The listing builds one solid part. Answer for the finished solid, in the listing's coordinates (mm). Face numbers are marked on the shaded views. A direction names the side the tool comes from. Give positions to 0.01 mm unless a question says otherwise; leave off trailing zeros. Order: outer loops, then holes, each group sorted by start corner. A loop starts at its lowest first (then second) coordinate and runs counter-clockwise, first axis right, second up.
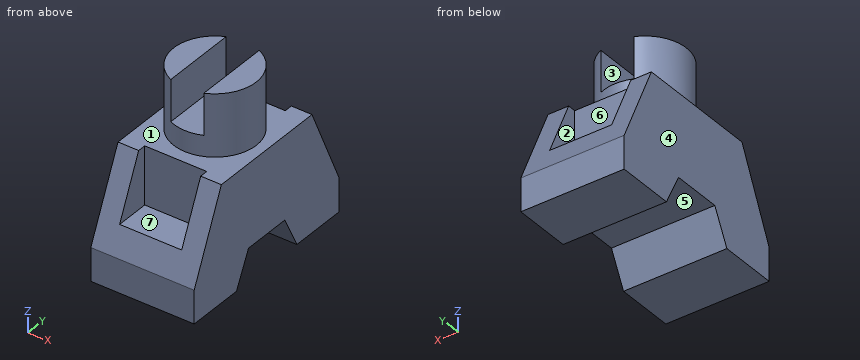
```python
from build123d import *

# Parameters (mm, degrees)
F0_W     = 9
F0_H     = 8
F0_W_2   = 5
F0_H_2   = 18
F0_W_3   = 10
F0_H_3   = 2
F1_DEPTH = 12.5
F2_R     = 10
F3_DEPTH = 15
F5_DEPTH = 10
F6_W     = 15
F6_H     = 8.3
F7_DEPTH = 14


with BuildPart() as f1:
    # F0 (on Right) → F1 (new body, symmetric)
    with BuildSketch(Plane.YZ):
        with Locations((-19.5, -10)):
            Rectangle(F0_W, F0_H)
        Polygon((-15, -6), (-15, -4), (-23.1, -4), (-24, -6), align=None)
        Polygon((-15, -4), (-15, 14), (-23.1, -4), align=None)
        with Locations((-12.5, 5)):
            Rectangle(F0_W_2, F0_H_2)
        with Locations((-7.5, 5)):
            Rectangle(F0_W_2, F0_H_2)
        with Locations((0, 5)):
            Rectangle(F0_W_3, F0_H_2)
        with Locations((7.5, 5)):
            Rectangle(F0_W_2, F0_H_2)
        with Locations((12.5, 5)):
            Rectangle(F0_W_2, F0_H_2)
        Polygon((23.1, -4), (15, 14), (15, -4), align=None)
        Polygon((23.1, -4), (15, -4), (15, -6), (24, -6), align=None)
        with Locations((19.5, -10)):
            Rectangle(F0_W, F0_H)
        with Locations((12.5, -10)):
            Rectangle(F0_W_2, F0_H)
        Polygon((10, -14), (10, -6), (6, -6), align=None)
        with Locations((12.5, -5)):
            Rectangle(F0_W_2, F0_H_3)
        with Locations((0, -5)):
            Rectangle(F0_W_3, F0_H_3)
        Polygon((-5, -6), (-5, -4), (-6, -6), align=None)
        Polygon((6, -6), (5, -4), (5, -6), align=None)
        Polygon((10, -6), (10, -4), (5, -4), (6, -6), align=None)
        Polygon((-6, -6), (-5, -4), (-10, -4), (-10, -6), align=None)
        Polygon((-10, -14), (-6, -6), (-10, -6), align=None)
        with Locations((-12.5, -10)):
            Rectangle(F0_W_2, F0_H)
        with Locations((-12.5, -5)):
            Rectangle(F0_W_2, F0_H_3)
    extrude(amount=F1_DEPTH, both=True)

    # F2 (on face) → F3 (join)
    with BuildSketch(Plane.XY.offset(14)):
        Circle(F2_R)
    extrude(amount=F3_DEPTH)

    # F4 (on face) → F5 (cut)
    with BuildSketch(Plane.XY.offset(29)):
        with BuildLine():
            ThreePointArc((4, 9.1651513899), (2.0430964369, 9.7890631293), (0, 10))
            ThreePointArc((0, 10), (-2.0430964369, 9.7890631293), (-4, 9.1651513899))
            Line((-4, 9.1651513899), (-4, -9.1651513899))
            ThreePointArc((-4, -9.1651513899), (-2.0430964369, -9.7890631293), (0, -10))
            ThreePointArc((0, -10), (2.0430964369, -9.7890631293), (4, -9.1651513899))
            Line((4, -9.1651513899), (4, 9.1651513899))
        make_face()
    extrude(amount=-F5_DEPTH, mode=Mode.SUBTRACT)

    # F6 (on Top) → F7 (cut)
    with BuildSketch(Plane.XY):
        with Locations((0, -17.15)):
            Rectangle(F6_W, F6_H)
        with Locations((0, 17.15)):
            Rectangle(F6_W, F6_H)
    extrude(amount=F7_DEPTH, mode=Mode.SUBTRACT)


solid = f1.part
```
1) Straight lines are drawn through the part: probe 1 along Z at (x, y) = (10.25, -11.5); probe 2 along Y at (x, z) = (2.5, -6.5); probe 3 along Y at (x, z) = (0.25, 5). For each, find the intervals that lie inside material, in ascending order.
Geometry says:
probe 1: z = -14 to 14
probe 2: y = -24 to -6.25, 6.25 to 24
probe 3: y = -13 to 13
2) Find section D-D (z = 26). Write down the section's boundary in (x, y).
Geometry says:
outline: (-4, -9.17) - (-4, 9.17) arc R10 ccw to start; (4, -9.17) arc R10 ccw to (4, 9.17) - close
3) For a pull along X with two mould halves and no side action, classify the marked faces 4, 5, 6 and 7 as +X half, -X half, draft (parallel to the pull), parting line (faces both ways), or undercut.
Geometry says:
face 4: -X half
face 5: draft
face 6: undercut
face 7: undercut
4) A tool of negligible diameter and unlimited length cuts with its end or side. For the marked faces 1, 2 and 3, from which of +Z, -Z, +X, -X, +Y, -Y can it reach the whole face along a straight path? Write none if from no direction.
Geometry says:
face 1: +Z
face 2: +Z, +Y
face 3: +Z, +Y, -Y
5) Given P1, Ø9.5, axis at x = 2, y = -3, coming from the -Z side; P2, Ø1, axis at y = -9, z = 20, coming from the +X side; P3, Ø2.5, axis at x = 0, y = -3.5, coming from the +Z side, each flat-ended and moving along its own axis, determine where each tip first touches the part or whether it passes through.
Geometry says:
P1: stops at z = -9.5
P2: stops at x = 5.27
P3: stops at z = 19
6) Find section C-C (x = 0). Write down the section's boundary in (y, z).
Geometry says:
outline: (-24, -14) - (-10, -14) - (-6, -6) - (6, -6) - (10, -14) - (24, -14) - (24, -6) - (21.3, 0) - (13, 0) - (13, 14) - (10, 14) - (10, 19) - (-10, 19) - (-10, 14) - (-13, 14) - (-13, 0) - (-21.3, 0) - (-24, -6) - close
7) Find section B-B (z = 10). Write down the section's boundary in (x, y), then the cut area to 3 significant figures.
Geometry says:
outline: (-12.5, -16.8) - (-7.5, -16.8) - (-7.5, -13) - (7.5, -13) - (7.5, -16.8) - (12.5, -16.8) - (12.5, 16.8) - (7.5, 16.8) - (7.5, 13) - (-7.5, 13) - (-7.5, 16.8) - (-12.5, 16.8) - close
area: 726 mm2
8) Find section A-A (y = 0). Write down the section's boundary in (x, z).
Geometry says:
outline: (-12.5, -6) - (12.5, -6) - (12.5, 14) - (10, 14) - (10, 29) - (4, 29) - (4, 19) - (-4, 19) - (-4, 29) - (-10, 29) - (-10, 14) - (-12.5, 14) - close
